```python
from build123d import *

# Parameters (mm, degrees)
F0_R     = 29.287505
F0_R_2   = 1
F1_DEPTH = 10
F4_W     = 4
F4_H     = 4
F4_R     = 1
F5_DEPTH = 2


# Not quite as in the source:
# - a fillet or chamfer that OpenCascade refuses, or shapes differently, is made with other operations: its cross-section is extruded or revolved along the edge and cut away or added


with BuildPart() as f1:
    # F0 (on Top) → F1 (new body)
    with BuildSketch(Plane.XY):
        Circle(F0_R)
        with Locations((-17.2713695087, -17.2713695087)):
            Circle(F0_R_2, mode=Mode.SUBTRACT)
        with Locations((0, -24.425405)):
            Circle(F0_R_2, mode=Mode.SUBTRACT)
        with Locations((-24.425405, 0)):
            Circle(F0_R_2, mode=Mode.SUBTRACT)
        with BuildLine():
            ThreePointArc((1.4936867141, 1.33), (0, -2), (-1.4936867141, 1.33))
            Line((-1.4936867141, 1.33), (1.4936867141, 1.33))
        make_face(mode=Mode.SUBTRACT)
        with Locations((17.2713695087, -17.2713695087)):
            Circle(F0_R_2, mode=Mode.SUBTRACT)
        with Locations((24.425405, 0)):
            Circle(F0_R_2, mode=Mode.SUBTRACT)
        with Locations((-17.2713695087, 17.2713695087)):
            Circle(F0_R_2, mode=Mode.SUBTRACT)
        with Locations((0, 24.425405)):
            Circle(F0_R_2, mode=Mode.SUBTRACT)
        with Locations((17.2713695087, 17.2713695087)):
            Circle(F0_R_2, mode=Mode.SUBTRACT)
    extrude(amount=F1_DEPTH)

    # F2: chamfer of 7.89245 x 4.55783 on 1 edges, made by hand

    # F2_s1 → F2_t2 (revolve, cut)
    with BuildSketch(Plane.XZ):
        Polygon((29.287505, 5.44217), (21.395055, 10), (29.287505, 10), align=None)
    revolve(axis=Axis((0, 0, 10), (0, 0, 1)), mode=Mode.SUBTRACT)

    # F4 (on offset) → F5 (cut)
    with BuildSketch(Plane.XY.offset(2)):
        with Locations((0, -24.425405)):
            Rectangle(F4_W, F4_H)
        with Locations((0, -24.425405)):
            Circle(F4_R, mode=Mode.SUBTRACT)
        Polygon((-20.0997966335, -17.2713695087), (-17.2713695087, -20.0997966335), (-14.442942384, -17.2713695087), (-17.2713695087, -14.442942384), align=None)
        Polygon((17.2713695087, -20.0997966335), (20.0997966335, -17.2713695087), (17.2713695087, -14.442942384), (14.442942384, -17.2713695087), align=None)
        with Locations((-24.425405, 0)):
            Rectangle(F4_W, F4_H)
        with Locations((24.425405, 0)):
            Rectangle(F4_W, F4_H)
        Polygon((-17.2713695087, 20.0997966335), (-20.0997966335, 17.2713695087), (-17.2713695087, 14.442942384), (-14.442942384, 17.2713695087), align=None)
        Polygon((20.0997966335, 17.2713695087), (17.2713695087, 20.0997966335), (14.442942384, 17.2713695087), (17.2713695087, 14.442942384), align=None)
        with Locations((0, 24.425405)):
            Rectangle(F4_W, F4_H)
        with Locations((0, -24.425405)):
            Circle(F4_R)
    extrude(amount=-F5_DEPTH, mode=Mode.SUBTRACT)


solid = f1.part
```
Here's how the part is built. I have some questions about the finished solid (model axes, mm). A direction names the side the tool comes from. Coordinates: 2 decimals unless noted, no trailing zeros. Write each loop counter-clockwise with the first axis right and the second up, starting at its lowest first coordinate (ties: lowest second). Pieces come first, ordered by that corner, then holes. Notation, with made-up numbers: (-35.5, 7.5) - (15.5, 7.5) arc R18 ccw to (15.5, 12.5) - close; hole circle Ø5 at (82.25, 2). An arc over 180 degrees is marked (long way). One line per item, written item: value.
1) We'd pull the mould along X, two halves only. Please class faces 1 (the flat face through (2, 24, 1)), 2 (the flat face through (6, 0, 0)): pulls with the +X half, pulls with the -X half, needs draft (parallel to the pull), parting line crosses it, or undercut.
Model answer:
face 1: undercut
face 2: needs draft
2) I'm going to push flat-ended pins straight in: P1, Ø1.6, axis at x = -0.5, z = 1, coming from the -Y side; P2, Ø0.6, axis at x = -0.5, z = 1.5, coming from the +Y side; P3, Ø1.6, axis at y = -25.5, z = 1.5, coming from the -X side. Where does each tip first touch, or does it pass through?
Model answer:
P1: stops at y = -29.29
P2: stops at y = 29.29
P3: stops at x = -15.74
3) I need wall thicknesses on line 1 along X through (y, z) = (-1.5, 1.25); line 2 along X through (y, z) = (-19, 0.75); line 3 along Y through (x, z) = (15, 1). Which ranges of each line are inside material? Lowest first, please.
Model answer:
line 1: x = -29.25 to -26.43, -22.43 to -1.32, 1.32 to 22.43, 26.43 to 29.25
line 2: x = -22.29 to -18.37, -16.17 to 16.17, 18.37 to 22.29
line 3: y = -25.15 to -17.83, -16.71 to 16.71, 17.83 to 25.15
4) Suppose I cut it at C-C on x = 0. Write out the boundary of the cut face in (y, z).
Model answer:
outline: (-29.29, 0) - (-26.43, 0) - (-26.43, 2) - (-25.43, 2) - (-25.43, 7.67) - (-29.29, 5.44) - close; (-23.43, 2) - (-22.43, 2) - (-22.43, 0) - (-2, 0) - (-2, 10) - (-21.4, 10) - (-23.43, 8.83) - close; (1.33, 0) - (22.43, 0) - (22.43, 2) - (23.43, 2) - (23.43, 8.83) - (21.4, 10) - (1.33, 10) - close; (25.43, 2) - (26.43, 2) - (26.43, 0) - (29.29, 0) - (29.29, 5.44) - (25.43, 7.67) - close
5) On a 3-axis mill with a long thin cutter (end or side, diameter ignored), from which of +Z, -Z, +X, -X, +Y, -Y can I reach the whole of each face in a straight line? I mean faces 3 (the cylindrical face through (-23.5, -0.38, 5.37)), 4 (the flat face through (-1, 25, 2)). Say none if no direction works.
Model answer:
face 3: +Z, -Z
face 4: -Z
6) Suppose I cut it at A-A on y = 0. Write out the boundary of the cut face in (x, z), and give its area (3 significant figures).
Model answer:
outline: (-29.29, 0) - (-26.43, 0) - (-26.43, 2) - (-25.43, 2) - (-25.43, 7.67) - (-29.29, 5.44) - close; (-23.43, 2) - (-22.43, 2) - (-22.43, 0) - (-2, 0) - (-2, 10) - (-21.4, 10) - (-23.43, 8.83) - close; (2, 0) - (22.43, 0) - (22.43, 2) - (23.43, 2) - (23.43, 8.83) - (21.4, 10) - (2, 10) - close; (25.43, 2) - (26.43, 2) - (26.43, 0) - (29.29, 0) - (29.29, 5.44) - (25.43, 7.67) - close
area: 469 mm²
7) Suppose I cut it at B-B on z = 3. State how many separate pieces and enclosed holes the cut face has, and give its area (3 significant figures).
Model answer:
separate pieces: 1
enclosed holes: 9
area: 2,660 mm²
